Autodesk Inventor part; units mm, degrees
ref_plane "YZ Plane" through (0, 0, 0) normal (1, 0, 0) x (0, 1, 0)
ref_plane "XZ Plane" through (0, 0, 0) normal (0, 1, 0) x (-1, 0, 0)
ref_plane "XY Plane" through (0, 0, 0) normal (0, 0, 1) x (1, 0, 0)
sketch "Sketch1" plane through (0, 0, 0) normal (0, 0, 1) x (1, 0, 0)
  line L0 (0, 0) -> (0, 50.8) construction
  line L1 (0, 0) -> (50.8, 0) construction
  line L2 (0, 50.8) -> (6.35, 50.8) construction
  line L3 (6.35, 50.8) -> (6.35, 0) construction
  line L4 (6.35, 50.8) -> (12.7, 50.8)
  line L5 (0, 25.6759) -> (14.9225, 25.6759) construction
  line L6 (12.7, 50.8) -> (14.9225, 25.6759)
  line L7 (0, 19.2751) -> (31.75, 19.2751) construction
  line L8 (31.75, 19.2751) -> (31.75, 25.6759)
  line L9 (14.9225, 25.6759) -> (31.75, 25.6759)
  line L10 (0, 9.5479) -> (15.8115, 9.5479) construction
  line L11 (31.75, 19.2751) -> (15.875, 19.2751)
  line L12 (15.875, 19.2751) -> (15.875, 6.5751)
  line L13 (15.875, 19.2751) -> (28.575, 19.2751) construction
  line L14 (0, 22.4755) -> (31.75, 22.4755) construction
  line L15 (6.35, 50.8) -> (6.35, 25.6759)
  line L16 (0, 6.5751) -> (8.2867, 6.5751) construction
  line L17 (8.2867, 6.5751) -> (15.875, 6.5751)
  line L18 (8.2867, 6.5751) -> (8.2867, 19.2751)
  line L19 (23.5585, 11.9908) -> (23.5585, 41.3472) construction
  line L20 (4.5974, 71.0633) -> (4.5974, -11.3243) construction
  line L21 (8.2867, 19.2751) -> (4.5974, 19.2751)
  line L22 (4.5974, 25.6759) -> (6.35, 25.6759)
  line L23 (4.5974, 25.6759) -> (4.5974, 19.2751)
  dimension "d2" = 50.8
  dimension "d3" = 90
  dimension "d4" = 6.35
  dimension "d5" = 6.35
  dimension "d6" = 14.9225
  dimension "d8" = 25.2222
  dimension "d9" = 31.75
  dimension "d11" = 6.4008
  dimension "d12" = 15.8115
  dimension "d13" = 12.7
  dimension "d14" = 90
  dimension "d15" = 8.2867
  dimension "d28" = 8.1915
  dimension "d55" = 4.5974
  dimension "d56" = 12.7
  dimension "d57" = 25.1241
revolve "Revolution1" add sketch "Sketch1" angle 360 about axis through (0, 0, 0) along (0, 1, 0)
fillet "Fillet1" radius 3.175 1 edges at (-14.9225, 25.6759, 0)
fillet "Fillet2" radius 3.175 1 edges at (-15.875, 19.2751, 0)
hole "Hole2" at (23.4944, 25.6759, -0.034) direction (0, -1, 0) diameter 5.3975 end through all
pattern_circular "Circular Pattern1" count 6 over 360 about axis through (0, 38.238, 0) along (0, -1, 0) of "Hole2"
sketch "Sketch2" plane through (0, 6.5751, 0) normal (0, -1, 0) x (1, 0, 0)
  circle A0 centre (0, 0) radius 8.2867 construction
  line L0 (-2.2055, 7.9879) -> (-2.2121, 9.8928)
  circle A1 centre (0, 0) radius 10.1371 construction
  line L1 (2.1506, 8.0028) -> (2.144, 9.9078)
  line L2 (-2.2055, 7.9879) -> (2.1506, 8.0028) construction
  arc A2 (2.144, 9.9078) -> (-2.2121, 9.8928) centre (0, 0) ccw
  arc A3 (2.1506, 8.0028) -> (-2.2055, 7.9879) centre (0, 0) ccw
  dimension "d43" = 1.905
  dimension "d44" = 4.3561
extrude "Extrusion1" cut sketch "Sketch2" against normal blind 12.7
pattern_circular "Circular Pattern2" count 6 over 360 about axis through (0, 12.9251, 0) along (0, -1, 0) of "Extrusion1"
sketch "Sketch3" plane through (0, 50.8, 0) normal (0, 1, 0) x (1, 0, 0)
  circle A0 centre (0, 0) radius 6.35 construction
  line L0 (0, 6.35) -> (0, 8.128) construction
  circle A1 centre (0, 0) radius 8.128 construction
  line L1 (-1.5685, 6.1532) -> (-2.0076, 7.8762)
  line L2 (1.5685, 6.1532) -> (2.0076, 7.8762)
  line L3 (-1.5685, 6.1532) -> (1.5685, 6.1532) construction
  arc A2 (2.0076, 7.8762) -> (-2.0076, 7.8762) centre (0, 0) ccw
  arc A3 (1.5685, 6.1532) -> (-1.5685, 6.1532) centre (0, 0) ccw
  dimension "d51" = 1.778
  dimension "d52" = 3.1369
extrude "Extrusion2" cut sketch "Sketch3" against normal blind 25.1206
properties part number "denso-6 coupler"
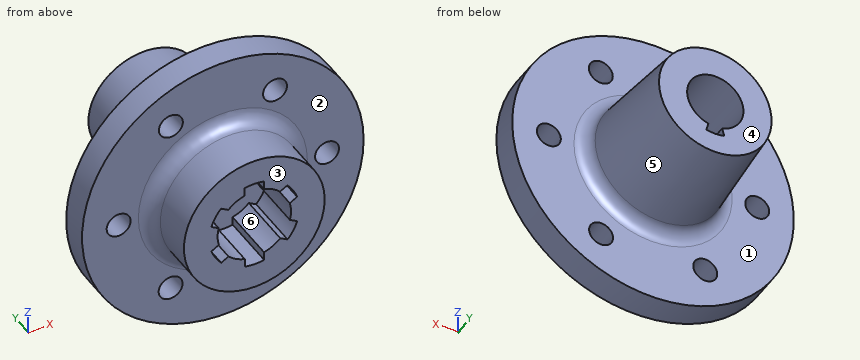
Here's how the part is built. I have some questions about the finished solid (model axes, mm). Face numbers are marked on the shaded views. A direction names the side the tool comes from. Coordinates: 2 decimals unless noted, no trailing zeros. Order: outer loops, then holes, each group sorted by start corner. A loop starts at its lowest first (then second) coordinate and runs counter-clockwise, first axis right, second up. Notation, with made-up numbers: M 18.5,31 L 47.5,31 A14 cw 47.5,57 Z; hole C 30,-37.5 d8. An arc over 180 degrees is marked long. Answer as a JSON object with one key per item and string values. Group by question number.
(1) Which directions (+Z, -Z, +X, -X, +Y, -Y) give clear straight access to the entire face, cutting with the end or side of a thin tool? Please do the marked faces 1, 2 and 3.
(2) Suppose I cut it at C-C, the plane z = 0. State how many separate pieces and enclosed holes the cut face has, then the cut area to 3 significant figures.
(3) Suppose I cut it at B-B, the plane y = 45. Please give me the cut outline in (x, z).
(4) If we mould it in two halves opening along X, with no side actions, what happens to the marked faces 4, 5 and 6? For each: released by +X, released by -X, zero draft, split by the parting line, or undercut.
(5) Suppose I cut it at D-D, the plane z = 24.5. Please give me the cut outline in (x, y), then the cut area to 3 significant figures.
(6) For pin 1 (8 mm diameter, centred on x = 10.5, z = -20.5, fed in from +Y); pin 2 (8 mm diameter, centred on x = 17, z = -22.5, fed in from -Y); pin 3 (4 mm diameter, centred on y = 31.5, z = -13.5, fed in from -X), each with a flat end and sliding along its axis, tell me the tip position at first contact or that it passes through.
(7) I need wall thicknesses on probe 1 along X at (y, z) = (23, 0); probe 2 along X at (y, z) = (23, -20); probe 3 along X at (y, z) = (19, -6). Which ranges of each line are inside material? Lowest first, please.
Values found:
{
 "1": {"face 1": "+Y", "face 2": "-Y", "face 3": "+Z, -Z, +X, -X, -Y"},
 "2": {"separate pieces": "4", "enclosed holes": "0", "area": "854 mm^2"},
 "3": {"outline": "C 0,0 d26.43; hole M -2.01,-7.88 A8.13 ccw 2.01,-7.88 L 1.57,-6.15 A6.35 ccw long -1.57,-6.15 Z"},
 "4": {"face 4": "zero draft", "face 5": "split by the parting line", "face 6": "undercut"},
 "5": {"outline": "M -20.19,19.28 L 20.19,19.28 L 20.19,25.68 L -20.19,25.68 Z", "area": "259 mm^2"},
 "6": {"pin 1": "stops at y = 25.68", "pin 2": "stops at y = 19.28", "pin 3": "stops at x = -8.69"},
 "7": {"probe 1": "x = -31.75 to -26.19, -20.8 to -4.6, 4.6 to 20.8, 26.19 to 31.75", "probe 2": "x = -24.66 to -14.46, -9.1 to 9.04, 14.39 to 24.66", "probe 3": "x = -16.71 to -8.17, -5.98 to -5.72, 5.72 to 6.09, 8.17 to 16.71"}
}
